Here's how the part is built. I have some questions about the finished solid (model axes, mm). A direction names the side the tool comes from. Give positions to 0.01 mm unless a question says otherwise; leave off trailing zeros. Write each loop counter-clockwise with the first axis right and the second up, starting at its lowest first coordinate (ties: lowest second). Pieces come first, ordered by that corner, then holes. Notation, with made-up numbers: (79.25, -39) -> (103.25, -39) arc R8 ccw to (103.25, -28) -> close; hole circle Ø4 at (60, 71). An arc over 180 degrees is marked (long way). Use one line per item in the form item = value.
```python
from build123d import *

# Parameters (mm, degrees)
CROQUIS1_W               = 76.5
CROQUIS1_H               = 40.7
SALIENTE_EXTRUIR1_DEPTH  = 2
CROQUIS2_W               = 2
CROQUIS2_H               = 5
CROQUIS2_W_2             = 5
CROQUIS2_H_2             = 2
SALIENTE_EXTRUIR2_DEPTH  = 33.3
CROQUIS3_W               = 12
CROQUIS3_H               = 2
SALIENTE_EXTRUIR3_DEPTH  = 12
NERVIO2_REACH            = 92.249
CROQUIS4_WALL_W          = 199.468346668
CROQUIS4_WALL_H          = 2
NERVIO7_REACH            = 82.33
CROQUIS5_WALL_W          = 179.62998513
CROQUIS5_WALL_H          = 2
NERVIO8_REACH            = 82.33
CROQUIS6_WALL_W          = 179.62998513
CROQUIS6_WALL_H          = 2
NERVIO9_REACH            = 92.249
CROQUIS7_WALL_W          = 199.468346668
CROQUIS7_WALL_H          = 2
CROQUIS8_R               = 1.75
CORTAR_EXTRUIR2_DEPTH    = 12
CROQUIS9_W               = 5
CROQUIS9_H               = 2
SALIENTE_EXTRUIR4_DEPTH  = 8
CROQUIS10_W              = 5
CROQUIS10_H              = 2
SALIENTE_EXTRUIR5_DEPTH  = 8
CROQUIS11_W              = 5
CROQUIS11_H              = 2
SALIENTE_EXTRUIR7_DEPTH  = 8
SALIENTE_EXTRUIR8_DEPTH  = 33.3
CORTAR_EXTRUIR5_START    = 8
CORTAR_EXTRUIR5_DEPTH    = 106.122924688
CORTAR_EXTRUIR6_DEPTH    = 22
CROQUIS15_W              = 2
CROQUIS15_H              = 2.7
CORTAR_EXTRUIR7_DEPTH    = 15
CROQUIS16_W              = 40.7
CROQUIS16_H              = 2
SALIENTE_EXTRUIR9_DEPTH  = 10
CROQUIS17_W              = 40.7
CROQUIS17_H              = 2
SALIENTE_EXTRUIR10_DEPTH = 10


with BuildPart() as part:
    # Croquis1 → Saliente-Extruir1 (new body)
    with BuildSketch(Plane(origin=(0, 0, 0), x_dir=(1, 0, 0), z_dir=(0, 1, 0))):
        Rectangle(CROQUIS1_W, CROQUIS1_H)
    extrude(amount=SALIENTE_EXTRUIR1_DEPTH)

    # Croquis2 → Saliente-Extruir2 (add)
    with BuildSketch(Plane(origin=(0, 2, 0), x_dir=(1, 0, 0), z_dir=(0, 1, 0))):
        Polygon((-36.25, -8.35), (-38.25, -8.35), (-38.25, -20.35), (-26.25, -20.35), (-26.25, -18.35), (-36.25, -18.35), align=None)
        with Locations((-37.25, 10.85)):
            Rectangle(CROQUIS2_W, CROQUIS2_H)
        with Locations((-28.75, 19.35)):
            Rectangle(CROQUIS2_W_2, CROQUIS2_H_2)
        with Locations((28.75, 19.35)):
            Rectangle(CROQUIS2_W_2, CROQUIS2_H_2)
        with Locations((37.25, 10.85)):
            Rectangle(CROQUIS2_W, CROQUIS2_H)
        Polygon((38.25, -20.35), (38.25, -8.35), (36.25, -8.35), (36.25, -18.35), (26.25, -18.35), (26.25, -20.35), align=None)
    extrude(amount=SALIENTE_EXTRUIR2_DEPTH)

    # Croquis3 → Saliente-Extruir3 (add)
    with BuildSketch(Plane.XY.offset(20.35)):
        with Locations((-32.25, 34.3)):
            Rectangle(CROQUIS3_W, CROQUIS3_H)
        with Locations((32.25, 34.3)):
            Rectangle(CROQUIS3_W, CROQUIS3_H)
    extrude(amount=SALIENTE_EXTRUIR3_DEPTH)

    # Croquis4 wall → Nervio2 (add, up to next)
    with BuildSketch(Plane(origin=(-38.25, 27.3, 26.35), x_dir=(0, -0.707106781187, -0.707106781187), z_dir=(0, -0.707106781187, 0.707106781187)), mode=Mode.PRIVATE) as nervio2_sk1:
        with Locations((0, 1)):
            Rectangle(CROQUIS4_WALL_W, CROQUIS4_WALL_H)
    nervio2_tool1 = extrude(nervio2_sk1.sketch, amount=-NERVIO2_REACH, mode=Mode.PRIVATE) - part.part
    add(nervio2_tool1.solids().sort_by_distance((-38.25, 27.3, 26.35))[0])

    # Croquis5 wall → Nervio7 (add, up to next)
    with BuildSketch(Plane(origin=(-26.25, 27.3, 26.35), x_dir=(0, -0.707106781187, -0.707106781187), z_dir=(0, 0.707106781187, -0.707106781187)), mode=Mode.PRIVATE) as nervio7_sk1:
        with Locations((0, 1)):
            Rectangle(CROQUIS5_WALL_W, CROQUIS5_WALL_H)
    nervio7_tool1 = extrude(nervio7_sk1.sketch, amount=NERVIO7_REACH, mode=Mode.PRIVATE) - part.part
    add(nervio7_tool1.solids().sort_by_distance((-26.25, 27.3, 26.35))[0])

    # Croquis6 wall → Nervio8 (add, up to next)
    with BuildSketch(Plane(origin=(26.25, 27.3, 26.35), x_dir=(0, -0.707106781187, -0.707106781187), z_dir=(0, -0.707106781187, 0.707106781187)), mode=Mode.PRIVATE) as nervio8_sk1:
        with Locations((0, 1)):
            Rectangle(CROQUIS6_WALL_W, CROQUIS6_WALL_H)
    nervio8_tool1 = extrude(nervio8_sk1.sketch, amount=-NERVIO8_REACH, mode=Mode.PRIVATE) - part.part
    add(nervio8_tool1.solids().sort_by_distance((26.25, 27.3, 26.35))[0])

    # Croquis7 wall → Nervio9 (add, up to next)
    with BuildSketch(Plane(origin=(38.25, 27.3, 26.35), x_dir=(0, -0.707106781187, -0.707106781187), z_dir=(0, 0.707106781187, -0.707106781187)), mode=Mode.PRIVATE) as nervio9_sk1:
        with Locations((0, 1)):
            Rectangle(CROQUIS7_WALL_W, CROQUIS7_WALL_H)
    nervio9_tool1 = extrude(nervio9_sk1.sketch, amount=NERVIO9_REACH, mode=Mode.PRIVATE) - part.part
    add(nervio9_tool1.solids().sort_by_distance((38.25, 27.3, 26.35))[0])

    # Croquis8 → Cortar-Extruir2 (cut)
    with BuildSketch(Plane(origin=(0, 35.3, 0), x_dir=(1, 0, 0), z_dir=(0, 1, 0))):
        with Locations(Location((-32.25, -26.35, 0), (0, 0, 270))):
            Circle(CROQUIS8_R)
        with Locations(Location((32.25, -26.35, 0), (0, 0, 270))):
            Circle(CROQUIS8_R)
    extrude(amount=-CORTAR_EXTRUIR2_DEPTH, mode=Mode.SUBTRACT)

    # Croquis9 → Saliente-Extruir4 (add)
    with BuildSketch(Plane(origin=(38.25, 0, 0), x_dir=(0, 0, -1), z_dir=(1, 0, 0))):
        with Locations((10.85, 34.3)):
            Rectangle(CROQUIS9_W, CROQUIS9_H)
    extrude(amount=SALIENTE_EXTRUIR4_DEPTH)

    # Croquis10 → Saliente-Extruir5 (add)
    with BuildSketch(Plane.ZY.offset(38.25)):
        with Locations((-10.85, 34.3)):
            Rectangle(CROQUIS10_W, CROQUIS10_H)
    extrude(amount=SALIENTE_EXTRUIR5_DEPTH)

    # Croquis11 → Saliente-Extruir7 (add)
    with BuildSketch(Plane(origin=(0, 0, -20.35), x_dir=(-1, 0, 0), z_dir=(0, 0, -1))):
        with Locations((-28.75, 34.3)):
            Rectangle(CROQUIS11_W, CROQUIS11_H)
        with Locations((28.75, 34.3)):
            Rectangle(CROQUIS11_W, CROQUIS11_H)
    extrude(amount=SALIENTE_EXTRUIR7_DEPTH)

    # Croquis13 → Saliente-Extruir8 (add)
    with BuildSketch(Plane(origin=(0, 2, 0), x_dir=(1, 0, 0), z_dir=(0, 1, 0))):
        Polygon((-38.25, 13.35), (-38.25, 20.35), (-31.25, 20.35), (-31.25, 18.35), (-36.25, 18.35), (-36.25, 13.35), align=None)
        Polygon((31.25, 20.35), (31.25, 18.35), (36.25, 18.35), (36.25, 13.35), (38.25, 13.35), (38.25, 20.35), align=None)
    extrude(amount=SALIENTE_EXTRUIR8_DEPTH)

    # Croquis12 → Cortar-Extruir5 (cut, through all)
    with BuildSketch(Plane.ZY.offset(38.25).offset(CORTAR_EXTRUIR5_START)):
        Polygon((-8.35, 32), (-8.35, 35.3), (-28.35, 35.3), (-28.35, 12), align=None)
    extrude(amount=-CORTAR_EXTRUIR5_DEPTH, mode=Mode.SUBTRACT)

    # Croquis14 → Cortar-Extruir6 (cut)
    with BuildSketch(Plane(origin=(0, 2, 0), x_dir=(1, 0, 0), z_dir=(0, 1, 0))):
        Polygon((-36.25, -13.35), (-38.25, -13.35), (-38.25, -20.35), (-31.25, -20.35), (-31.25, -18.35), (-36.25, -18.35), align=None)
        Polygon((31.25, -18.35), (31.25, -20.35), (38.25, -20.35), (38.25, -13.35), (36.25, -13.35), (36.25, -18.35), align=None)
    extrude(amount=CORTAR_EXTRUIR6_DEPTH, mode=Mode.SUBTRACT)

    # Croquis15 → Cortar-Extruir7 (cut)
    with BuildSketch(Plane.XY.offset(20.35)):
        with Locations((-37.25, 22.65)):
            Rectangle(CROQUIS15_W, CROQUIS15_H)
        with Locations((37.25, 22.65)):
            Rectangle(CROQUIS15_W, CROQUIS15_H)
    extrude(amount=CORTAR_EXTRUIR7_DEPTH, mode=Mode.SUBTRACT)

    # Croquis16 → Saliente-Extruir9 (add)
    with BuildSketch(Plane.ZY.offset(38.25)):
        with Locations((0, 1)):
            Rectangle(CROQUIS16_W, CROQUIS16_H)
    extrude(amount=SALIENTE_EXTRUIR9_DEPTH)

    # Croquis17 → Saliente-Extruir10 (add)
    with BuildSketch(Plane(origin=(38.25, 0, 0), x_dir=(0, 0, -1), z_dir=(1, 0, 0))):
        with Locations((0, 1)):
            Rectangle(CROQUIS17_W, CROQUIS17_H)
    extrude(amount=SALIENTE_EXTRUIR10_DEPTH)


solid = part.part
```
Q1. I want a section at D-D, the plane y = 26. Write out the boundary of the cut face in (x, z), and give its area (3 significant figures).
Result set:
outline = (-38.25, -14.35) -> (-36.25, -14.35) -> (-36.25, -8.35) -> (-38.25, -8.35) -> close; (-38.25, 8.35) -> (-36.25, 8.35) -> (-36.25, 18.35) -> (-26.25, 18.35) -> (-26.25, 25.05) -> (-28.25, 25.05) -> (-28.25, 20.35) -> (-36.25, 20.35) -> (-36.25, 25.05) -> (-38.25, 25.05) -> close; (26.25, 18.35) -> (36.25, 18.35) -> (36.25, 8.35) -> (38.25, 8.35) -> (38.25, 25.05) -> (36.25, 25.05) -> (36.25, 20.35) -> (28.25, 20.35) -> (28.25, 25.05) -> (26.25, 25.05) -> close; (36.25, -14.35) -> (38.25, -14.35) -> (38.25, -8.35) -> (36.25, -8.35) -> close
area = 150 mm2
Q2. I want a section at C-C, the plane z = 26.35. Write out the boundary of the cut face in (x, y).
Result set:
outline = (-38.25, 27.3) -> (-36.25, 27.3) -> (-36.25, 33.3) -> (-34, 33.3) -> (-34, 35.3) -> (-38.25, 35.3) -> close; (-30.5, 33.3) -> (-28.25, 33.3) -> (-28.25, 27.3) -> (-26.25, 27.3) -> (-26.25, 35.3) -> (-30.5, 35.3) -> close; (26.25, 27.3) -> (28.25, 27.3) -> (28.25, 33.3) -> (30.5, 33.3) -> (30.5, 35.3) -> (26.25, 35.3) -> close; (34, 33.3) -> (36.25, 33.3) -> (36.25, 27.3) -> (38.25, 27.3) -> (38.25, 35.3) -> (34, 35.3) -> close
Q3. Will these pins go through, and if not, where does the flat tip stop? pin 1 Ø11 at (y, z) = (21.5, 25.5) entering from +X; pin 2 Ø0.6 at (y, z) = (8, 19.5) entering from +X; pin 3 Ø1.6 at (x, y) = (37.5, 22.5) entering from -Z.
Result set:
pin_1 = 38.25
pin_2 = 31.25
pin_3 = -18.65
Q4. If I drill on line 1 along X through (y, z) = (34.25, 26.35); line 2 along X through (y, z) = (28, 13); line 3 along Z through (x, y) = (32, 34), over which ranges is the centre line in solid material (lowest first)? Write a range as from..to.
Result set:
line_1 = -38.25..-34, -30.5..-26.25, 26.25..30.5, 34..38.25
line_2 = -38.25..-36.25, 36.25..38.25
line_3 = 18.35..24.62, 28.08..32.35
Q5. I want a section at B-B, the plane x = 32.25. Write out the boundary of the cut face in (y, z), and give its area (3 significant figures).
Result set:
outline = (0, -20.35) -> (20, -20.35) -> (22, -18.35) -> (2, -18.35) -> (2, 20.35) -> (0, 20.35) -> close; (24, 18.35) -> (35.3, 18.35) -> (35.3, 24.6) -> (33.3, 24.6) -> (33.3, 20.35) -> (24, 20.35) -> close; (33.3, 28.1) -> (35.3, 28.1) -> (35.3, 32.35) -> (33.3, 32.35) -> close
area = 159 mm2
Q6. Which directions (+Z, -Z, +X, -X, +Y, -Y) give clear straight access to the entire face, cutting with the end or side of a thin tool? Please do faces 4 (the face through (-36.25, 22, 12)), 5 (the face through (31.25, 13, 19)), 6 (the face through (37, 18, 8.35)), 7 (the face through (-26.25, 26, 23)).
Result set:
face_4 = +Y
face_5 = +Z, +X
face_6 = +X, -X, +Y
face_7 = +Z, -Z, +Y
Q7. If we mould it in two halves opening along Z, with no side actions, what happens to faces 1 (the face through (-30, 22, 18.35)), 2 (the face through (-38.25, 26, 15)), 3 (the face through (-37.24, 28.72, 27.77))? For each: +Z half, -Z half, draft (parallel to the pull), parting line (faces both ways), or undercut.
Result set:
face_1 = undercut
face_2 = draft
face_3 = +Z half
Q8. I want a section at A-A, the plane y = 19. Write out the boundary of the cut face in (x, z), and give its area (3 significant figures).
Result set:
outline = (-38.25, -20.35) -> (-26.25, -20.35) -> (-26.25, -18.35) -> (-36.25, -18.35) -> (-36.25, -8.35) -> (-38.25, -8.35) -> close; (-38.25, 8.35) -> (-36.25, 8.35) -> (-36.25, 13.35) -> (-38.25, 13.35) -> close; (-31.25, 18.35) -> (-26.25, 18.35) -> (-26.25, 20.35) -> (-31.25, 20.35) -> close; (26.25, -20.35) -> (38.25, -20.35) -> (38.25, -8.35) -> (36.25, -8.35) -> (36.25, -18.35) -> (26.25, -18.35) -> close; (26.25, 18.35) -> (31.25, 18.35) -> (31.25, 20.35) -> (26.25, 20.35) -> close; (36.25, 8.35) -> (38.25, 8.35) -> (38.25, 13.35) -> (36.25, 13.35) -> close
area = 128 mm2
